Design review of the part built by this model. Coordinates are the model's own, in mm. A direction names the side the tool comes from. Coordinates: 2 decimals unless noted, no trailing zeros. Order: outer loops, then holes, each group sorted by start corner. A loop starts at its lowest first (then second) coordinate and runs counter-clockwise, first axis right, second up. Notation, with made-up numbers: M 20.25,33.5 L 36.25,33.5 A18 cw 36.25,49.5 Z; hole C 10.5,-39.5 d9. An arc over 180 degrees is marked long. Answer as a JSON object with one key per item and string values.
from build123d import *

# Parameters (mm, degrees)
SOCKET_1_SKETCH_W = 15
SOCKET_1_SKETCH_H = 5.5


with BuildPart() as part:
    # NPT_Ext_30 Sketch → NPT_Ext_30 (revolve)
    with BuildSketch(Plane.XY, mode=Mode.PRIVATE) as npt_ext_30_sk:
        Polygon((12.7, 0), (12.7, 5.5), (0, 5.5), (0, 9), (-30, 9), (-30, 0), align=None)
    revolve(npt_ext_30_sk.sketch.rotate(Axis((-1000, 0, 0), (1, 0, 0)), 90), axis=Axis((-1000, 0, 0), (1, 0, 0)))

    # Socket 1 Sketch → Socket 1 (revolve, cut)
    with BuildSketch(Plane.XY, mode=Mode.PRIVATE) as socket_1_sk:
        with Locations((-23.5, 2.75)):
            Rectangle(SOCKET_1_SKETCH_W, SOCKET_1_SKETCH_H)
    revolve(socket_1_sk.sketch.rotate(Axis((-1000, 0, 0), (1, 0, 0)), 90), axis=Axis((-1000, 0, 0), (1, 0, 0)), mode=Mode.SUBTRACT)


solid = part.part
1) Add section A-A (z = 0). State the section outline as (x, y) points, and give its area (3 significant figures).
Taken from the geometry:
{"outline": "M -30,-9 L 0,-9 L 0,-5.5 L 12.7,-5.5 L 12.7,5.5 L 0,5.5 L 0,9 L -30,9 L -30,5.5 L -16,5.5 L -16,-5.5 L -30,-5.5 Z", "area": "526 mm2"}
2) Add section C-C (x = -23). State the section outline as (y, z) points.
Taken from the geometry:
{"outline": "C 0,0 d18; hole C 0,0 d11"}
3) To check wall thickness, follow L1, parallel to Y at x = -21.5, z = 0; L2, parallel to Z at x = -20, y = -0.25; L3, parallel to X at y = 1.5, z = -0.75. State the ranges of each line that lie inside material, in increasing order.
Taken from the geometry:
{"L1": "y = -9 to -5.5, 5.5 to 9", "L2": "z = -9 to -5.49, 5.49 to 9", "L3": "x = -16 to 12.7"}
4) Insertion check: pin 1 Ø6 at (x, y) = (3.5, 1.5) entering from -Z; pin 2 Ø1 at (x, y) = (-7, -3.5) entering from -Z; pin 3 Ø1.5 at (x, y) = (-23.5, 3.5) entering from -Z. Each pin has a flat end and moves straight along its axis. Give the tip position at first contact, or say it passes through.
Taken from the geometry:
{"pin 1": "stops at z = -5.5", "pin 2": "stops at z = -8.49", "pin 3": "stops at z = -8.57"}
5) Tool access review of faces 1 (the cylindrical face through (6.26, 5.37, -1.19)), 2 (the cylindrical face through (-15.21, -6.083, -6.633)), 3 (the cylindrical face through (-22.9, 5.37, -1.19)): name each direction out of +Z, -Z, +X, -X, +Y, -Y from which nothing blocks a thin tool from reaching the whole face with its end or side.
Taken from the geometry:
{"face 1": "+X", "face 2": "+X, -X", "face 3": "-X"}
6) Add section D-D (x = -13). State the section outline as (y, z) points, and give its area (3 significant figures).
Taken from the geometry:
{"outline": "C 0,0 d18", "area": "254 mm2"}
